Build history of the part. All positions in model axes, mm. A direction names the side the tool comes from. Give positions to 0.01 mm unless a question says otherwise; leave off trailing zeros. Write each loop counter-clockwise with the first axis right and the second up, starting at its lowest first coordinate (ties: lowest second). Pieces come first, ordered by that corner, then holes. Notation, with made-up numbers: M -5.75,22.5 L 37.25,22.5 A14 cw 37.25,38.5 Z; hole C 37.25,-36 d10. An arc over 180 degrees is marked long. Return JSON: item names as keys, results as strings. Group by question number.
Q1. Band-saw the part on A-A, the plane z = 51. Give the cut face in (x, y), then the cut area to 3 significant figures.
Q2. Wall check: probe 1 along Z at (x, y) = (22, 15); probe 2 along X at (y, z) = (0.95, 64.36); probe 3 along Y at (x, z) = (10.25, 22). Give the ranges that are in metal, low to high.
Q3. Flat gauge pins, fed straight in: pin 1 Ø0.9 at (x, y) = (7, 31.5) entering from +Z; pin 2 Ø2.5 at (y, z) = (27.77, 65.18) entering from -X. Where does each tip first touch, or does it go through?
Q4. Tool access for faces 3 (the flat face through (12, 30, 15)), 4 (the flat face through (21.929, 26, 78)), 5 (the flat face through (8.836, 31.479, 10.521)), 6 (the flat face through (15.943, 3.521, 62.839)), 7 (the flat face through (23, 18, 76.36)): list every direction of +Z, -Z, +X, -X, +Y, -Y with a clear straight run to the whole face (end or side of a thin tool).
Q5. Pull direction Y, two halves, no side cores. Call faces 1 (the flat face through (3.64, 31.48, 10.48)), 2 (the flat face through (6, 4, 39)): +Y half, -Y half, draft (parallel to the pull), parting line (faces both ways), or undercut.
Q6. Band-saw the part on B-B, the plane y = 12. Give the cut face in (x, z), then the cut area to 3 significant figures.
from build123d import *

# Parameters (mm, degrees)
EXTRUDE_1_DEPTH     = 30
EXTRUDE_2_DEPTH     = 3
CUT_EXTRUDE_1_DEPTH = 3
CUT_EXTRUDE_START   = -17
SKETCH_4_R          = 1.65
CUT_EXTRUDE_2_DEPTH = 76
CUT_EXTRUDE_3_DEPTH = 3
FILLET_1_R          = 5
EXTRUDE_3_DEPTH     = 49.36
EXTRUDE_4_DEPTH     = 3
CUT_EXTRUDE_4_DEPTH = 3
SKETCH_10_R         = 1.5
CUT_EXTRUDE_5_DEPTH = 12
FILLET_2_R          = 5
CUT_EXTRUDE_6_DEPTH = 3
SKETCH_12_R         = 1.65
CUT_EXTRUDE_7_DEPTH = 15


with BuildPart() as part:
    # Sketch 1 → Extrude 1 (new body)
    with BuildSketch(Plane.XY):
        Polygon((0, 0), (30, 0), (30, 35), (0, 35), (0, 30), (25, 30), (25, 5), (0, 5), align=None)
    extrude(amount=EXTRUDE_1_DEPTH)

    # Sketch 2 → Extrude 2 (add)
    with BuildSketch(Plane.XY.offset(30)):
        with BuildLine():
            Line((12.5, 30), (25, 30))
            Line((25, 30), (25, 5))
            Line((25, 5), (12.5, 5))
            ThreePointArc((12.5, 5), (21.929285786, 17.5), (12.5, 30))
        make_face()
    extrude_2 = extrude(amount=-EXTRUDE_2_DEPTH)

    # Mirror 1: Extrude 2 across plane
    add(extrude_2.mirror(Plane.XY.offset(15)))

    # Sketch 3 → Cut-Extrude 1 (cut)
    with BuildSketch(Plane(origin=(0, 5, 0), x_dir=(1, 0, 0), z_dir=(0, 1, 0))):
        Polygon((4.517949192, -24), (2.785898385, -21), (4.517949192, -18), (7.982050808, -18), (9.714101615, -21), (7.982050808, -24), align=None)
        Polygon((2.785898385, -9), (4.517949192, -12), (7.982050808, -12), (9.714101615, -9), (7.982050808, -6), (4.517949192, -6), align=None)
    extrude(amount=-CUT_EXTRUDE_1_DEPTH, mode=Mode.SUBTRACT)

    # Sketch 4 → Cut-Extrude 2 (cut)
    with BuildSketch(Plane(origin=(0, 2, 0), x_dir=(1, 0, 0), z_dir=(0, 1, 0)).offset(CUT_EXTRUDE_START)):
        with Locations(Location((6.25, -21, 0), (0, 0, 90))):
            Circle(SKETCH_4_R)
    cut_extrude_2 = extrude(amount=CUT_EXTRUDE_2_DEPTH, mode=Mode.SUBTRACT)

    # Mirror 2: Cut-Extrude 2 across plane
    add(cut_extrude_2.mirror(Plane.XY.offset(15)), mode=Mode.SUBTRACT)

    # Sketch 5 → Cut-Extrude 3 (cut)
    with BuildSketch(Plane.XZ.offset(-30)):
        Polygon((9.714101615, 21), (7.982050808, 24), (4.517949192, 24), (2.785898385, 21), (4.517949192, 18), (7.982050808, 18), align=None)
    cut_extrude_3 = extrude(amount=-CUT_EXTRUDE_3_DEPTH, mode=Mode.SUBTRACT)

    # Mirror 3: Cut-Extrude 3 across plane
    add(cut_extrude_3.mirror(Plane.XY.offset(15)), mode=Mode.SUBTRACT)

    # Fillet 1
    fillet_1_edges = [part.edges().sort_by_distance(p)[0] for p in [
        (0, 2.5, 0),
        (0, 32.5, 30),
        (0, 32.5, 0),
    ]]
    fillet(fillet_1_edges, radius=FILLET_1_R)

    # Sketch 7 → Extrude 3 (add)
    with BuildSketch(Plane.XY.offset(30)):
        Polygon((0, 0), (30, 0), (30, 35), (25, 35), (25, 5), (0, 5), align=None)
    extrude(amount=EXTRUDE_3_DEPTH)

    # Sketch 8 → Extrude 4 (add)
    with BuildSketch(Plane.XY.offset(79.36)):
        with BuildLine():
            Line((21.929285786, 17.5), (21.929285786, 35))
            Line((21.929285786, 35), (25, 35))
            Line((25, 35), (25, 5))
            Line((25, 5), (12.5, 5))
            ThreePointArc((12.5, 5), (19.307611392, 9.67118415), (21.929285786, 17.5))
        make_face()
    extrude(amount=-EXTRUDE_4_DEPTH)

    # Sketch 9 → Cut-Extrude 4 (cut)
    with BuildSketch(Plane.ZY.offset(-25)):
        Polygon((65.18, 31.229416542), (62.18, 29.497365734), (62.18, 26.033264119), (65.18, 24.301213312), (68.18, 26.033264119), (68.18, 29.497365734), align=None)
        Polygon((41.18, 15.698786688), (38.18, 13.966735881), (38.18, 10.502634266), (41.18, 8.770583458), (44.18, 10.502634266), (44.18, 13.966735881), align=None)
    extrude(amount=-CUT_EXTRUDE_4_DEPTH, mode=Mode.SUBTRACT)

    # Sketch 10 → Cut-Extrude 5 (cut)
    with BuildSketch(Plane.ZY.offset(-28)):
        with Locations(Location((41.18, 12.234685073, 0), (0, 0, 270))):
            Circle(SKETCH_10_R)
        with Locations(Location((65.18, 27.765314927, 0), (0, 0, 270))):
            Circle(SKETCH_10_R)
    extrude(amount=-CUT_EXTRUDE_5_DEPTH, mode=Mode.SUBTRACT)

    # Fillet 2
    fillet_2_edges = [part.edges().sort_by_distance(p)[0] for p in [
        (0, 2.5, 79.36),
    ]]
    fillet(fillet_2_edges, radius=FILLET_2_R)

    # Sketch 11 → Cut-Extrude 6 (cut)
    with BuildSketch(Plane(origin=(0, 5, 0), x_dir=(1, 0, 0), z_dir=(0, 1, 0))):
        Polygon((15.064802613, -64.36), (16.79685342, -67.36), (20.260955035, -67.36), (21.993005843, -64.36), (20.260955035, -61.36), (16.79685342, -61.36), align=None)
        Polygon((9.935197387, -42), (8.20314658, -39), (4.739044965, -39), (3.006994157, -42), (4.739044965, -45), (8.20314658, -45), align=None)
    extrude(amount=-CUT_EXTRUDE_6_DEPTH, mode=Mode.SUBTRACT)

    # Sketch 12 → Cut-Extrude 7 (cut)
    with BuildSketch(Plane(origin=(0, 2, 0), x_dir=(1, 0, 0), z_dir=(0, 1, 0))):
        with Locations(Location((6.471095772, -42, 0), (0, 0, 270))):
            Circle(SKETCH_12_R)
        with Locations(Location((18.528904228, -64.36, 0), (0, 0, 270))):
            Circle(SKETCH_12_R)
    extrude(amount=-CUT_EXTRUDE_7_DEPTH, mode=Mode.SUBTRACT)


solid = part.part
From the geometry:
{
 "1": {"outline": "M 0,0 L 30,0 L 30,35 L 25,35 L 25,5 L 0,5 Z", "area": "300 mm^2"},
 "2": {"probe 1": "z = 0 to 3, 27 to 30, 76.36 to 79.36", "probe 2": "x = 0 to 16.88, 20.18 to 30", "probe 3": "y = 0 to 5, 30 to 35"},
 "3": {"pin 1": "stops at z = 30", "pin 2": "passes through"},
 "4": {"face 3": "-X", "face 4": "+Z, -X, +Y", "face 5": "none", "face 6": "+Y", "face 7": "-X, +Y"},
 "5": {"face 1": "undercut", "face 2": "draft"},
 "6": {"outline": "M 20.71,0 L 30,0 L 30,39.7 L 28,39.7 L 28,38.18 L 25,38.18 L 25,30 L 20.71,30 L 20.71,27 L 25,27 L 25,3 L 20.71,3 Z; M 20.71,76.36 L 25,76.36 L 25,44.18 L 28,44.18 L 28,42.66 L 30,42.66 L 30,79.36 L 20.71,79.36 Z", "area": "411 mm^2"}
}
